Model file for the job. Use its own axes, mm. Face numbers are marked on the shaded views. A direction names the side the tool comes from. Round coordinates to 2 decimals unless told otherwise and drop trailing zeros. Order: outer loops, then holes, each group sorted by start corner. A loop starts at its lowest first (then second) coordinate and runs counter-clockwise, first axis right, second up. Notation, with made-up numbers: (-10, -26.75) - (46, -26.75) arc R27 ccw to (46, -2.75) - close; hole circle Ø10 at (-34, -37). An arc over 180 degrees is marked (long way). Answer as CSV lines item,"result". Start each with the question number.
1. Band-saw the part on D-D on y = -17.5. List the corners of the cut face in (x, z), then the cut area to 3 significant figures.
2. Pull direction Y, two halves, no side cores. Call the marked faces 1, 2 and 3: released by +Y, released by -Y, zero draft, split by the parting line, or undercut.
3. Wall check: line 1 along Y through (x, z) = (2.6, 6); line 2 along Y through (x, z) = (2.15, 24); line 3 along Y through (x, z) = (2.2, 0). Give the ranges that are in metal, low to high. Write a range as [from, to].
4. 3-axis set-ups, long thin cutter, end or side, ignore diameter. For the marked faces 4 and 5: which of +Z, -Z, +X, -X, +Y, -Y reach the whole face in a straight line?
5. Band-saw the part on B-B on y = 0. State how many separate pieces and enclosed holes the cut face has, then the cut area to 3 significant figures.
6. Band-saw the part on A-A on z = 0. List the corners of the cut face in (x, y), then the cut area to 3 significant figures.
7. Pin check, flat tips, straight feed: pin 1 Ø6.5 at (y, z) = (0, 0) entering from -X; pin 2 Ø4 at (y, z) = (8, 16.5) entering from +X; pin 3 Ø4 at (y, z) = (-0.5, 27.5) entering from +X; pin 4 Ø1.5 at (x, z) = (2.5, 13.5) entering from -Y. Stop position of each tip, or through.
8. Band-saw the part on C-C on z = -20.5. List the corners of the cut face in (x, y), then the cut area to 3 significant figures.
```python
from build123d import *

# Parameters (mm, degrees)
CROQUIS2_R                                  = 3.5
CROQUIS2_R_2                                = 1.5
CORTAR_EXTRUIR1_DEPTH                       = 4
CORTAR_EXTRUIR2_DEPTH                       = 10
CORTAR_EXTRUIR3_START                       = -2.5
CORTAR_EXTRUIR3_DEPTH                       = 2.5
CORTAR_EXTRUIR4_DEPTH                       = 2
CROQUIS7_R                                  = 2.75
CROQUIS7_R_2                                = 3.25
CORTAR_EXTRUIR6_DEPTH                       = 2.5
AVELLANADO_PARA_TORNILLO_CON_CABEZA_2_COUNT = 2
AVELLANADO_PARA_TORNILLO_CON_CABEZA_2_PITCH = 17


with BuildPart() as part:
    # Croquis1 → Revolución1 (revolve)
    with BuildSketch(Plane.XY, mode=Mode.PRIVATE) as revoluci_n1_sk:
        Polygon((0, 0), (4, 0), (4, 9.5), (1.5, 9.5), (1.5, 22.5), (4, 22.5), (4, 32.5), (0, 32.5), align=None)
    revolve(revoluci_n1_sk.sketch.rotate(Axis((0, 0, 0), (1, 0, 0)), 90), axis=Axis((0, 0, 0), (1, 0, 0)))

    # Croquis2 → Cortar-Extruir1 (cut)
    with BuildSketch(Plane(origin=(4, 0, 0), x_dir=(0, 0, -1), z_dir=(1, 0, 0))):
        Circle(CROQUIS2_R)
        with Locations((25.406687144, -10.52379439)):
            Circle(CROQUIS2_R_2)
        with Locations((10.52379439, -25.406687144)):
            Circle(CROQUIS2_R_2)
        with Locations((-10.52379439, -25.406687144)):
            Circle(CROQUIS2_R_2)
        with Locations((-25.406687144, -10.52379439)):
            Circle(CROQUIS2_R_2)
        with Locations((-25.406687144, 10.52379439)):
            Circle(CROQUIS2_R_2)
        with Locations((25.406687144, 10.52379439)):
            Circle(CROQUIS2_R_2)
    extrude(amount=-CORTAR_EXTRUIR1_DEPTH, mode=Mode.SUBTRACT)

    # Croquis3 → Cortar-Extruir2 (cut)
    with BuildSketch(Plane(origin=(4, 0, 0), x_dir=(0, 0, -1), z_dir=(1, 0, 0))):
        with BuildLine():
            Line((-22.980970389, 22.980970389), (-15.909902577, 15.909902577))
            ThreePointArc((-15.909902577, 15.909902577), (0, 22.5), (15.909902577, 15.909902577))
            Line((15.909902577, 15.909902577), (22.980970389, 22.980970389))
            ThreePointArc((22.980970389, 22.980970389), (0, 32.5), (-22.980970389, 22.980970389))
        make_face()
    extrude(amount=-CORTAR_EXTRUIR2_DEPTH, mode=Mode.SUBTRACT)

    # Croquis4 → Cortar-Extruir3 (cut)
    with BuildSketch(Plane(origin=(4, 0, 0), x_dir=(0, 0, -1), z_dir=(1, 0, 0)).offset(CORTAR_EXTRUIR3_START)):
        with BuildLine():
            Line((2.832561639, -32.376327688), (2.266049311, -25.90106215))
            ThreePointArc((2.266049311, -25.90106215), (0, -26), (-2.266049311, -25.90106215))
            Line((-2.266049311, -25.90106215), (-2.832561639, -32.376327688))
            ThreePointArc((-2.832561639, -32.376327688), (0, -32.5), (2.832561639, -32.376327688))
        make_face()
    extrude(amount=CORTAR_EXTRUIR3_DEPTH, mode=Mode.SUBTRACT)

    # Croquis5 → Cortar-Extruir4 (cut)
    with BuildSketch(Plane(origin=(4, 0, 0), x_dir=(0, 0, -1), z_dir=(1, 0, 0))):
        with BuildLine():
            ThreePointArc((31.625, 0), (27.5, 4.125), (23.375, 0))
            Line((23.375, 0), (31.625, 0))
        make_face()
        with BuildLine():
            Line((31.625, 0), (23.375, 0))
            ThreePointArc((23.375, 0), (27.5, -4.125), (31.625, 0))
        make_face()
        with BuildLine():
            ThreePointArc((-31.625, 0), (-27.5, -4.125), (-23.375, 0))
            Line((-23.375, 0), (-31.625, 0))
        make_face()
        with BuildLine():
            Line((-31.625, 0), (-23.375, 0))
            ThreePointArc((-23.375, 0), (-27.5, 4.125), (-31.625, 0))
        make_face()
    extrude(amount=-CORTAR_EXTRUIR4_DEPTH, mode=Mode.SUBTRACT)

    # Croquis7 → Cortar-Extruir6 (cut)
    with BuildSketch(Plane(origin=(4, 0, 0), x_dir=(0, 0, -1), z_dir=(1, 0, 0))):
        with Locations((8.5, 0)):
            Circle(CROQUIS7_R)
        with Locations((-8.5, 0)):
            Circle(CROQUIS7_R)
        with Locations((25.406687144, -10.52379439)):
            Circle(CROQUIS7_R_2)
        with Locations((10.52379439, -25.406687144)):
            Circle(CROQUIS7_R_2)
        with Locations((-10.52379439, -25.406687144)):
            Circle(CROQUIS7_R_2)
        with Locations((-25.406687144, -10.52379439)):
            Circle(CROQUIS7_R_2)
        with Locations((-25.406687144, 10.52379439)):
            Circle(CROQUIS7_R_2)
        with Locations((25.406687144, 10.52379439)):
            Circle(CROQUIS7_R_2)
    extrude(amount=-CORTAR_EXTRUIR6_DEPTH, mode=Mode.SUBTRACT)

    # Croquis10 → Avellanado para tornillo con cabeza ovalada de #31 (revolve, cut)
    with BuildSketch(Plane(origin=(1.5, 0, 8.5), x_dir=(0, 0, -1), z_dir=(0, 1, 0))):
        Polygon((0, 0), (0, 1.5), (1.397, 1.5), (1.397, 1.300261411), (2.5273, 0), align=None)
    avellanado_para_tornillo_con_cabeza_oval = revolve(axis=Axis((7.85, 0, 8.5), (-1, 0, 0)), mode=Mode.SUBTRACT)

    # Avellanado para tornillo con cabeza  2: Avellanado para tornillo con cabeza ovalada de #31 ×2
    with Locations(*[(0, 0, -i * AVELLANADO_PARA_TORNILLO_CON_CABEZA_2_PITCH) for i in range(1, AVELLANADO_PARA_TORNILLO_CON_CABEZA_2_COUNT)]):
        add(avellanado_para_tornillo_con_cabeza_oval, mode=Mode.SUBTRACT)


solid = part.part
```
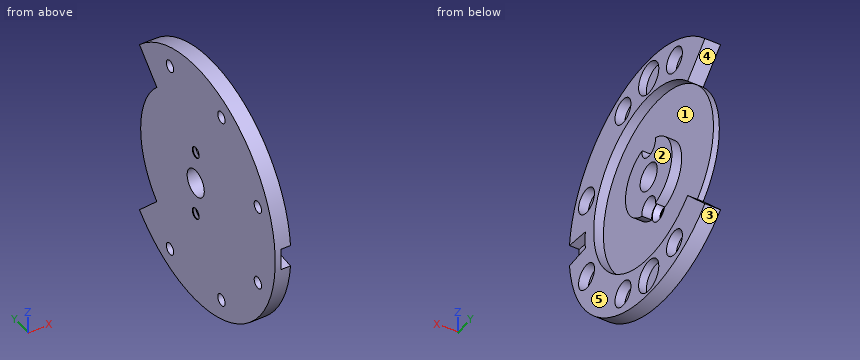
Reply:
1,outline,"(0, -27.39) - (4, -27.39) - (4, -14.14) - (1.5, -14.14) - (1.5, 14.14) - (4, 14.14) - (4, 27.39) - (0, 27.39) - close"
1,area,"148 mm2"
2,face 1,"undercut"
2,face 2,"zero draft"
2,face 3,"split by the parting line"
3,line 1,"y = [-31.94, -21.69], [-7.37, -1.15], [1.15, 7.37]"
3,line 2,"y = [-21.91, -13.45], [-7.59, -2.18], [2.18, 7.59], [13.45, 21.91]"
3,line 3,"y = [-26, -22.5], [-9.5, -3.5], [3.5, 9.5]"
4,face 4,"+X, -X, +Y"
4,face 5,"+Z, -Z, +X, +Y, -Y"
5,separate pieces,"4"
5,enclosed holes,"0"
5,area,"104 mm2"
6,outline,"(0, -32.5) - (1.5, -32.5) - (1.5, -26) - (4, -26) - (4, -22.5) - (1.5, -22.5) - (1.5, -9.5) - (4, -9.5) - (4, -3.5) - (0, -3.5) - close; (0, 3.5) - (4, 3.5) - (4, 9.5) - (1.5, 9.5) - (1.5, 22.5) - (0, 22.5) - close"
6,area,"111 mm2"
7,pin 1,"passes through"
7,pin 2,"stops at x = 1.5"
7,pin 3,"stops at x = 2"
7,pin 4,"stops at y = -29.89"
8,outline,"(0, -25.22) - (4, -25.22) - (4, -9.27) - (1.5, -9.27) - (1.5, 9.27) - (4, 9.27) - (4, 20.5) - (0, 20.5) - close"
8,area,"137 mm2"
